from build123d import *
from build123d.topology import SkipClean

# Parameters (mm, degrees)
SKETCH1_R           = 6
SKETCH1_R_2         = 5
BOSS_EXTRUDE1_DEPTH = 60
FILLET1_R           = 10
FILLET2_R           = 9
CIRPATTERN1_COUNT   = 3


with BuildPart() as part:
    # Sketch1 → Boss-Extrude1 (new body)
    with BuildSketch(Plane.XY):
        with BuildLine():
            ThreePointArc((7.496526573, -11.545), (30.821844121, -17.795), (13.746526573, -0.719682453))
            Line((13.746526573, -0.719682453), (6.25, 12.264682453))
            ThreePointArc((6.25, 12.264682453), (0, 35.59), (-6.25, 12.264682453))
            Line((-6.25, 12.264682453), (-13.746526573, -0.719682453))
            ThreePointArc((-13.746526573, -0.719682453), (-30.821844121, -17.795), (-7.496526573, -11.545))
            Line((-7.496526573, -11.545), (7.496526573, -11.545))
        make_face()
        with Locations((19.996526573, -11.545)):
            Circle(SKETCH1_R, mode=Mode.SUBTRACT)
        with Locations((0, 23.09)):
            Circle(SKETCH1_R, mode=Mode.SUBTRACT)
        Circle(SKETCH1_R_2, mode=Mode.SUBTRACT)
        with Locations((-19.996526573, -11.545)):
            Circle(SKETCH1_R, mode=Mode.SUBTRACT)
    extrude(amount=BOSS_EXTRUDE1_DEPTH)

    # Fillet1
    # the kernel refuses this fillet: 10 mm, written as the material it adds along each edge
    with BuildSketch(Plane(origin=(13.746526573, -0.719682453, 0), x_dir=(0.9572887202141619, 0.28913371673108657, 0), z_dir=(0, 0, 1))) as fillet1_piece_1:
        with BuildLine():
            CenterArc((7.988652571, 9.736032088), FILLET1_R, 193.193899981, 63.612200039)
            Line((-1.747379517, 7.453559925), (0, 0))
            ThreePointArc((0, 0), (2.853090204, 0.32995989), (5.706180408, 0))
        make_face()
    extrude(amount=60)
    with BuildSketch(Plane(origin=(6.25, 12.264682453, 0), x_dir=(0.4999999999999975, -0.86602540378444, 0), z_dir=(0, 0, 1))) as fillet1_piece_2:
        with BuildLine():
            CenterArc((7.655644371, 10), FILLET1_R, 206.387799961, 63.612200039)
            ThreePointArc((-1.302419794, 5.555555556), (-0.32995989, 2.853090204), (0, 0))
            Line((0, 0), (7.655644371, 0))
        make_face()
    extrude(amount=60)

    # Fillet2
    fillet2_edges = [part.edges().sort_by_distance(p)[0] for p in [
        (7.496526573, -11.545, 30),
        (-7.496526573, -11.545, 30),
        (-13.746526573, -0.719682453, 30),
        (-6.25, 12.264682453, 30),
    ]]
    fillet(fillet2_edges, radius=FILLET2_R)

    # Sketch2 → Revolve3 (revolve)
    with BuildSketch(Plane(origin=(0, 0, 0), x_dir=(0, 0, -1), z_dir=(1, 0, 0)), mode=Mode.PRIVATE) as revolve3_sk:
        with BuildLine():
            Line((-60, 35.59), (-60, 29.09))
            Line((-60, 29.09), (-65, 29.09))
            Line((-65, 29.09), (-65, 41.59))
            ThreePointArc((-65, 41.59), (-62.102636282, 38.921136432), (-60, 35.59))
        make_face()
    revolve3 = revolve(revolve3_sk.sketch.rotate(Axis((0, 23.09, 60), (0, 0, -1)), 90), axis=Axis((0, 23.09, 60), (0, 0, -1)))

    # CirPattern1: Revolve3 ×3 about axis
    with SkipClean():  # the faces are left unmerged after this step: merging them gives an invalid solid
        cirpattern1_axis = Axis((0, 0, 0), (0, 0, 1))
        for i in range(1, CIRPATTERN1_COUNT):
            add(revolve3.rotate(cirpattern1_axis, i * 360 / CIRPATTERN1_COUNT))

    # Mirror1: Revolve3 across plane
    with SkipClean():  # the faces are left unmerged after this step: merging them gives an invalid solid
        add(revolve3.mirror(Plane.XY.offset(30)))

    # Mirror1 copy 1 sketch → Mirror1 copy 1 (revolve)
    with SkipClean():  # the faces are left unmerged after this step: merging them gives an invalid solid
        with BuildSketch(Plane(origin=(0, 0, 60), x_dir=(0, 0, 1), z_dir=(-0.4999999999999998, 0.8660254037844387, 0))):
            with BuildLine():
                Line((-60, -35.59), (-60, -29.09))
                Line((-60, -29.09), (-65, -29.09))
                Line((-65, -29.09), (-65, -41.59))
                ThreePointArc((-65, -41.59), (-62.102636282, -38.921136432), (-60, -35.59))
            make_face()
        revolve(axis=Axis((-19.996526573, -11.545, 0), (0, 0, -1)))

    # Mirror1 copy 2 sketch → Mirror1 copy 2 (revolve)
    with SkipClean():  # the faces are left unmerged after this step: merging them gives an invalid solid
        with BuildSketch(Plane(origin=(0, 0, 60), x_dir=(0, 0, 1), z_dir=(-0.5000000000000004, -0.8660254037844384, 0))):
            with BuildLine():
                Line((-60, -35.59), (-60, -29.09))
                Line((-60, -29.09), (-65, -29.09))
                Line((-65, -29.09), (-65, -41.59))
                ThreePointArc((-65, -41.59), (-62.102636282, -38.921136432), (-60, -35.59))
            make_face()
        revolve(axis=Axis((19.996526573, -11.545, 0), (0, 0, -1)))


solid = part.part
The model under review builds one solid part; all positions refer to its coordinate system, in mm. A direction names the side the tool comes from. Give positions to 0.01 mm unless a question says otherwise; leave off trailing zeros. Write each loop counter-clockwise with the first axis right and the second up, starting at its lowest first coordinate (ties: lowest second). Pieces come first, ordered by that corner, then holes. Notation, with made-up numbers: M 24.25,-4.75 L 30.25,-4.75 A21 cw 30.25,6.25 Z; hole C -28,35.25 d4. An arc over 180 degrees is marked long. One line per question, with ' | ' between items. Start each with the question number.
Item 1: Wall thickness on line 1 (Z direction, x = -8.5, y = 12.5); line 2 (X direction, y = 23.09, z = 21); line 3 (X direction, y = -15.5, z = 24.5): over which ranges is each line inside the solid? List them lowest first. Write a range as from..to.
Item 2: For faces 1 (the cylindrical face through (-13.826, 1.906, 30.42)), 2 (the cylindrical face through (5.38, -13, 30.42)), 3 (the flat face through (4.4, 18.7, -5)), 4 (the cylindrical face through (8.75, 11.11, 29.58)), list the 3-axis set-ups (+Z, -Z, +X, -X, +Y, -Y) from which the entire face can be reached by the end or side of a thin tool; tool diameter is ignored.
Item 3: We need section B-B on y = 9. Give the number of separate pieces and of enclosed holes in the cut face, plus the area to 3 significant figures.
Item 4: For pin 1 (15.5 mm diameter, centred on x = 20, y = -11.55, fed in from +Z); pin 2 (3 mm diameter, centred on x = -15, z = 20, fed in from +Y); pin 3 (10 mm diameter, centred on y = 26, z = 44, fed in from +X); pin 4 (10 mm diameter, centred on y = -0.5, z = 52, fed in from +X), all flat-tipped, find the tip position at first contact; note any pin that passes through.
Item 5: We need section A-A on z = 29. Write out the cut boundary in (x, y) (1 decimal), plus the area to 3 significant figures.
Item 6: Draft analysis for pull direction X (two halves, no side actions). For faces 5 (the cylindrical face through (-8.57, 11.16, 30.42)), 6 (the cylindrical face through (-5.38, -13, 30.42)), 7 (the flat face through (4.4, 18.7, 65)), state which applies: released by +X, released by -X, zero draft, split by the parting line, or undercut.
Results found:
1) line 1: z = -5..-0.55, 0..60, 60.55..65 | line 2: x = -12.5..-6, 6..12.5 | line 3: x = -31.85..-24.51, -15.48..-7.92, 7.92..15.48, 24.51..31.85
2) face 1: none | face 2: -Y | face 3: -Z, +X, -X, +Y, -Y | face 4: +X
3) separate pieces: 3 | enclosed holes: 0 | area: 1,200 mm2
4) pin 1: stops at z = 65 | pin 2: stops at y = 2.09 | pin 3: stops at x = 12.5 | pin 4: stops at x = 30.94
5) outline: M -18.9,0.9 A12.5 ccw long -8.6,-16.8 A9 cw -0.5,-11.5 L 0.5,-11.5 A9 cw 8.6,-16.8 A12.5 ccw long 19.2,0.9 A10 cw 10,5.8 A10 cw 10.4,16.2 A12.5 ccw long -10.2,15.9 A9 cw -9.8,6.2 L -10.2,5.4 A9 cw Z; hole C -20,-11.5 d12; hole C 0,23.1 d12; hole C 0,0 d10; hole C 20,-11.5 d12 | area: 1,550 mm2
6) face 5: released by -X | face 6: undercut | face 7: zero draft
